The model under review builds one solid part; all positions refer to its coordinate system, in mm. Face numbers are marked on the shaded views. A direction names the side the tool comes from. Give positions to 0.01 mm unless a question says otherwise; leave off trailing zeros. Write each loop counter-clockwise with the first axis right and the second up, starting at its lowest first coordinate (ties: lowest second). Pieces come first, ordered by that corner, then holes.
from build123d import *

# Parameters (mm, degrees)
SKETCH2_W             = 140
SKETCH2_H             = 15
BASE_DEPTH            = 15
SKETCH3_R             = 7.5
CENTER_CUT_DEPTH      = 142.598022585
SKETCH4_W             = 1
SKETCH4_H             = 25.4
ANTENNA_PCB_DEPTH     = 10.2
SKETCH11_W            = 3.5
SKETCH11_H            = 15
COAX_CONNECTOR_DEPTH  = 5
LENS_START            = -23.9
SKETCH8_R             = 9
LENS_DEPTH            = 8.6
FILLET1_R             = 4.8
SKETCH17_W            = 82.5
SKETCH17_H            = 3
CUT_EXTRUDE4_DEPTH    = 2
SKETCH19_W            = 4
SKETCH19_H            = 5.2
CUT_EXTRUDE5_DEPTH    = 5.8
SKETCH21_W            = 3.5
SKETCH21_H            = 4.5
CUT_EXTRUDE6_DEPTH    = 15
FILLET7_SIZE          = 1.5
COAX_CABLE_HOLE_START = -2
COAX_CABLE_HOLE_DEPTH = 2
SKETCH23_W            = 12.7
SKETCH23_H            = 7.5
CUT_EXTRUDE7_DEPTH    = 10
BOSS_EXTRUDE1_REACH   = 143.598
CUT_EXTRUDE10_DEPTH   = 2.7
SKETCH31_R            = 2.65
MOUNTING_HOLES_DEPTH  = 5
FILLET11_SIZE         = 2
PHOTODIODE_PCB_START  = -62.8
SKETCH10_W            = 25.4
SKETCH10_H            = 20.4
PHOTODIODE_PCB_DEPTH  = 1
CUT_EXTRUDE13_DEPTH   = 5
CHAMFER2_SIZE         = 3
FILTER_MOUNT_START    = -56.1
FILTER_MOUNT_DEPTH    = 6.7
FILTER_SPACE_START    = -58
SKETCH36_R            = 7
FILTER_SPACE_DEPTH    = 1.5


# Some blends are built 0.0001 mm under size
with BuildPart() as part:
    # Sketch2 → Base (new body)
    with BuildSketch(Plane(origin=(0, 0, 0), x_dir=(1, 0, 0), z_dir=(0, 1, 0))):
        with Locations((70, -7.5)):
            Rectangle(SKETCH2_W, SKETCH2_H)
        with Locations((70, 7.5)):
            Rectangle(SKETCH2_W, SKETCH2_H)
    extrude(amount=-BASE_DEPTH)

    # Sketch3 → Center_cut (cut, through all)
    with BuildSketch(Plane.ZY):
        Circle(SKETCH3_R)
    extrude(amount=-CENTER_CUT_DEPTH, mode=Mode.SUBTRACT)

    # Sketch4 → Antenna_PCB (cut)
    with BuildSketch(Plane(origin=(0, 0, 0), x_dir=(1, 0, 0), z_dir=(0, 1, 0))):
        with Locations((0.5, 0)):
            Rectangle(SKETCH4_W, SKETCH4_H)
    extrude(amount=-ANTENNA_PCB_DEPTH, mode=Mode.SUBTRACT)

    # Sketch11 → Coax_connector (cut)
    with BuildSketch(Plane.ZY.offset(-1)):
        with Locations((-10.95, 0)):
            Rectangle(SKETCH11_W, SKETCH11_H)
    extrude(amount=-COAX_CONNECTOR_DEPTH, mode=Mode.SUBTRACT)

    # Sketch8 → Lens (cut)
    with BuildSketch(Plane.ZY.offset(-1).offset(LENS_START)):
        Circle(SKETCH8_R)
    extrude(amount=-LENS_DEPTH, mode=Mode.SUBTRACT)

    # Fillet1
    fillet1_edges = [part.edges().sort_by_distance(p)[0] for p in [
        (70, -15, -15),
        (70, -15, 15),
    ]]
    fillet(fillet1_edges, radius=FILLET1_R)

    # Sketch17 → Cut-Extrude4 (cut)
    with BuildSketch(Plane(origin=(0, 0, -15), x_dir=(-1, 0, 0), z_dir=(0, 0, -1))):
        with Locations((-44.75, -8.7)):
            Rectangle(SKETCH17_W, SKETCH17_H)
    extrude(amount=-CUT_EXTRUDE4_DEPTH, mode=Mode.SUBTRACT)

    # Sketch19 → Cut-Extrude5 (cut)
    with BuildSketch(Plane(origin=(0, 0, -15), x_dir=(-1, 0, 0), z_dir=(0, 0, -1))):
        with Locations((-5.5, -7.6)):
            Rectangle(SKETCH19_W, SKETCH19_H)
    extrude(amount=-CUT_EXTRUDE5_DEPTH, mode=Mode.SUBTRACT)

    # Sketch21 → Cut-Extrude6 (cut)
    with BuildSketch(Plane(origin=(0, 0, -15), x_dir=(-1, 0, 0), z_dir=(0, 0, -1))):
        with Locations((-84.25, -6.45)):
            Rectangle(SKETCH21_W, SKETCH21_H)
    extrude(amount=-CUT_EXTRUDE6_DEPTH, mode=Mode.SUBTRACT)

    # Fillet7
    fillet7_edges = [part.edges().sort_by_distance(p)[0] for p in [
        (84.25, -8.7, -13),
    ]]
    chamfer(fillet7_edges, length=FILLET7_SIZE - 0.0001)  # a hair under: the kernel refuses the full size

    # Sketch22 → Coax_cable_hole (add)
    with BuildSketch(Plane(origin=(140, 0, 0), x_dir=(0, 0, -1), z_dir=(1, 0, 0)).offset(COAX_CABLE_HOLE_START)):
        with BuildLine():
            ThreePointArc((-7.5, 0), (0, -7.5), (7.5, 0))
            Line((7.5, 0), (3.25, 0))
            ThreePointArc((3.25, 0), (0, -3.25), (-3.25, 0))
            Line((-3.25, 0), (-7.5, 0))
        make_face()
        with BuildLine():
            Line((11.25, -8), (11.25, 0))
            Line((11.25, 0), (7.5, 0))
            ThreePointArc((7.5, 0), (0, -7.5), (-7.5, 0))
            Line((-7.5, 0), (-11.25, 0))
            Line((-11.25, 0), (-11.25, -8))
            Line((-11.25, -8), (11.25, -8))
        make_face()
    extrude(amount=COAX_CABLE_HOLE_DEPTH)

    # Sketch23 → Cut-Extrude7 (cut)
    with BuildSketch(Plane.ZY.offset(-1)):
        with Locations((6.35, -3.75)):
            Rectangle(SKETCH23_W, SKETCH23_H)
    extrude(amount=-CUT_EXTRUDE7_DEPTH, mode=Mode.SUBTRACT)

    # Sketch24 → Boss-Extrude1 (add, up to next)
    with BuildSketch(Plane(origin=(0, 0, 0), x_dir=(1, 0, 0), z_dir=(0, 1, 0)), mode=Mode.PRIVATE) as boss_extrude1_sk1:
        Polygon((1, -12.7), (11, -8.455251838), (11, -12.7), align=None)
    boss_extrude1_tool1 = extrude(boss_extrude1_sk1.sketch, amount=-BOSS_EXTRUDE1_REACH, mode=Mode.PRIVATE) - part.part
    add(boss_extrude1_tool1.solids().sort_by_distance((7.666667, 0, 11.285084))[0])

    # Sketch27 → Cut-Extrude10 (cut)
    with BuildSketch(Plane(origin=(0, -7.5, 0), x_dir=(1, 0, 0), z_dir=(0, 1, 0))):
        Polygon((10.687415097, -7.718847955), (11, -8.455251838), (11, -7.586163536), align=None)
        Polygon((1, -12.7), (11, -8.455251838), (10.687415097, -7.718847955), (1, -11.830911698), align=None)
    extrude(amount=-CUT_EXTRUDE10_DEPTH, mode=Mode.SUBTRACT)

    # Sketch31 → Mounting_holes (cut)
    with BuildSketch(Plane(origin=(0, 0, 0), x_dir=(1, 0, 0), z_dir=(0, 1, 0))):
        with Locations(Location((17.95, -11.25, 0), (0, 0, 270))):
            Circle(SKETCH31_R)
        with Locations(Location((122, -11.25, 0), (0, 0, 270))):
            Circle(SKETCH31_R)
        with Locations(Location((122, 11.25, 0), (0, 0, 90))):
            Circle(SKETCH31_R)
        with Locations(Location((17.95, 11.25, 0), (0, 0, 90))):
            Circle(SKETCH31_R)
        with Locations(Location((69.975, -11.25, 0), (0, 0, 270))):
            Circle(SKETCH31_R)
        with Locations(Location((69.975, 11.25, 0), (0, 0, 90))):
            Circle(SKETCH31_R)
    extrude(amount=-MOUNTING_HOLES_DEPTH, mode=Mode.SUBTRACT)

    # Fillet11
    fillet11_edges = [part.edges().sort_by_distance(p)[0] for p in [
        (7.5, -8.7, -13),
        (3.5, -7.5, -10.95),
    ]]
    chamfer(fillet11_edges, length=FILLET11_SIZE)

    # Sketch10 → Photodiode_PCB (cut)
    with BuildSketch(Plane.ZY.offset(-1).offset(PHOTODIODE_PCB_START)):
        Rectangle(SKETCH10_W, SKETCH10_H)
    extrude(amount=-PHOTODIODE_PCB_DEPTH, mode=Mode.SUBTRACT)

    # Sketch33 → Cut-Extrude13 (cut)
    with BuildSketch(Plane.ZY.offset(-64.8)):
        with BuildLine():
            Line((-2.5, -10.2), (0, -10.2))
            Line((0, -10.2), (0, -7.5))
            ThreePointArc((0, -7.5), (-1.26826484, -7.391989197), (-2.5, -7.071067812))
            Line((-2.5, -7.071067812), (-2.5, -10.2))
        make_face()
        with BuildLine():
            Line((0, -10.2), (2.5, -10.2))
            Line((2.5, -10.2), (2.5, -7.071067812))
            ThreePointArc((2.5, -7.071067812), (1.26826484, -7.391989197), (0, -7.5))
            Line((0, -7.5), (0, -10.2))
        make_face()
    extrude(amount=-CUT_EXTRUDE13_DEPTH, mode=Mode.SUBTRACT)

    # Chamfer2
    # the kernel refuses this chamfer: 3 mm, written as the material it takes off along each edge
    with BuildSketch(Plane(origin=(69.8, 0, 0), x_dir=(0, -0.2008336879156208, 0.9796253517535216), z_dir=(0, 0.9796253517535216, 0.2008336879156208))) as chamfer2_piece_1_section:
        Polygon((7.5, CHAMFER2_SIZE), (7.5 + CHAMFER2_SIZE, 0), (7.5, 0), align=None)
    chamfer2_piece_1 = revolve(axis=Axis((69.8, 0, 0), (1, 0, 0)), revolution_arc=156.828569884, mode=Mode.PRIVATE)
    chamfer2_piece_1 = split(chamfer2_piece_1, bisect_by=Plane(origin=(70.802116042, -8.337432159, -2.5), z_dir=(0, 0, 1)), keep=Keep.TOP, mode=Mode.PRIVATE)
    chamfer2_piece_1 = split(chamfer2_piece_1, bisect_by=Plane(origin=(70.802116042, -10.2, 0), z_dir=(0, 1, 0)), keep=Keep.TOP, mode=Mode.PRIVATE)
    chamfer2_piece_1 = split(chamfer2_piece_1, bisect_by=Plane(origin=(70.802116042, -8.337432159, 2.5), z_dir=(0, 0, -1)), keep=Keep.TOP, mode=Mode.PRIVATE)
    add(chamfer2_piece_1, mode=Mode.SUBTRACT)

    # Sketch35 → Filter_mount (add)
    with BuildSketch(Plane.ZY.offset(-1).offset(FILTER_MOUNT_START)):
        with BuildLine():
            Line((-5, 0), (-7.5, 0))
            ThreePointArc((-7.5, 0), (-5.303300859, -5.303300859), (0, -7.5))
            ThreePointArc((0, -7.5), (5.303300859, -5.303300859), (7.5, 0))
            Line((7.5, 0), (5, 0))
            ThreePointArc((5, 0), (0, -5), (-5, 0))
        make_face()
    extrude(amount=-FILTER_MOUNT_DEPTH)

    # Sketch36 → Filter_space (cut)
    with BuildSketch(Plane.ZY.offset(-1).offset(FILTER_SPACE_START)):
        Circle(SKETCH36_R)
    extrude(amount=-FILTER_SPACE_DEPTH, mode=Mode.SUBTRACT)


solid = part.part
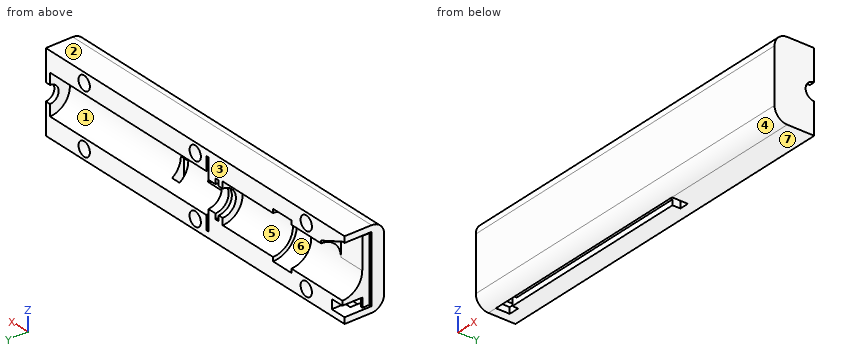
1) To check wall thickness, follow probe 1 along X at (y, z) = (-1.3, -11.25) (3 decimals); probe 2 along X at (y, z) = (-6.25, 2.25); probe 3 along X at (y, z) = (-7, -6). State the ranges of each line that lie inside material, in increasing order.
2) Consider section A-A, the plane x = 46. Give the boundary of the cut face in (y, z).
3) Consider section C-C, the plane y = -12. Give the boundary of the cut face in (x, z).
4) The part is to be moulded in two halves that separate along Z. For the marked faces 1, 2, 3 and 4, say which applies: +Z half, -Z half, draft (parallel to the pull), parting line (faces both ways), or undercut.
5) Insertion check: pin 1 (3 mm diameter, centred on y = -3, z = -5.5, fed in from -X); pin 2 (3 mm diameter, centred on x = 105, y = -12, fed in from -Z); pin 3 (1.6 mm diameter, centred on x = 19, z = 11, fed in from +Y). Each pin has a flat end and moves straight along its axis. Give the tip position at first contact, or say it passes through.
6) Tool access review of the marked faces 5, 6 and 7: name each direction out of +Z, -Z, +X, -X, +Y, -Y from which nothing blocks a thin tool from reaching the whole face with its end or side.
7) Consider section B-B, the plane x = 117.5. Give the boundary of the cut face in (y, z), then the cut area to 3 significant figures.
Answer block:
1. probe 1: x = 6 to 15.3, 20.6 to 63.8, 64.8 to 67.325, 72.625 to 119.35, 124.65 to 140
1. probe 2: x = 57.1 to 59, 60.5 to 63.8, 138 to 140
1. probe 3: x = 1 to 63.8, 64.8 to 82.5, 86 to 140
2. outline: (-15, -10.2) arc R4.8 ccw to (-10.2, -15) - (-10.2, -13) - (-7.2, -13) - (-7.2, -15) - (0, -15) - (0, -7.5) arc R7.5 cw to (0, 7.5) - (0, 15) - (-10.2, 15) arc R4.8 ccw to (-15, 10.2) - close
3. outline: (0, -14.65) - (140, -14.65) - (140, 14.65) - (0, 14.65) - close
4. face 1: undercut
4. face 2: +Z half
4. face 3: draft
4. face 4: -Z half
5. pin 1: stops at x = 1
5. pin 2: stops at z = -14.99
5. pin 3: stops at y = -5
6. face 5: -X, +Y
6. face 6: +Y
6. face 7: -Z, +X, -X, +Y, -Y
7. outline: (-15, -10.2) arc R4.8 ccw to (-10.2, -15) - (0, -15) - (0, -7.5) arc R7.5 cw to (0, 7.5) - (0, 15) - (-10.2, 15) arc R4.8 ccw to (-15, 10.2) - close
7. area: 352 mm2
